Study the drawing (mm; zero at the part's minimum x, y, z) and answer. Give positions to 0.01 mm unless a question says otherwise; leave off trailing zeros. Order: outer loops, then holes, each group sorted by start corner. A loop starts at its lowest first (then second) coordinate and runs counter-clockwise, first axis right, second up. Notation, with made-up numbers: (55.5, -2.5) - (99.5, -2.5) arc R32 cw to (99.5, 31.5) - close; hole circle Ø4 at (-5, -7). An arc over 180 degrees is marked (long way). Write each question's results on one line, items separated by ' | '. Start each with the question number.
1. Determine the mould class of the marked faces 1, 2 and 3 for opening direction X: released by +X, released by -X, zero draft, split by the parting line, or undercut.
2. Section C-C (z = 9.5) is taken. Give the vertices of the cut face in (x, y), and give its area (3 significant figures).
3. Find the intervals of material crossed by L1, parallel to Y at x = 6, z = 9.4; L2, parallel to Y at x = 6, z = 6; L3, parallel to Z at x = 8, y = 8.5, in increasing order.
4. Section D-D (x = 3.75) is taken. Give the vertices of the cut face in (y, z).
5. Section B-B (x = 6) is taken. Give the vertices of the cut face in (y, z).
6. Section A-A (y = 6) is taken. Give the vertices of the cut face in (x, z), and give its area (3 significant figures).
7. Flat-ended cylindrical pins translate along their axes: pin 1 (1 mm diameter, centred on x = 4.5, z = 6, fed in from -Y); pin 2 (1.5 mm diameter, centred on x = 7, y = 6, fed in from -Z). Find the tip coordinate at first contact, or state that the pin passes through.
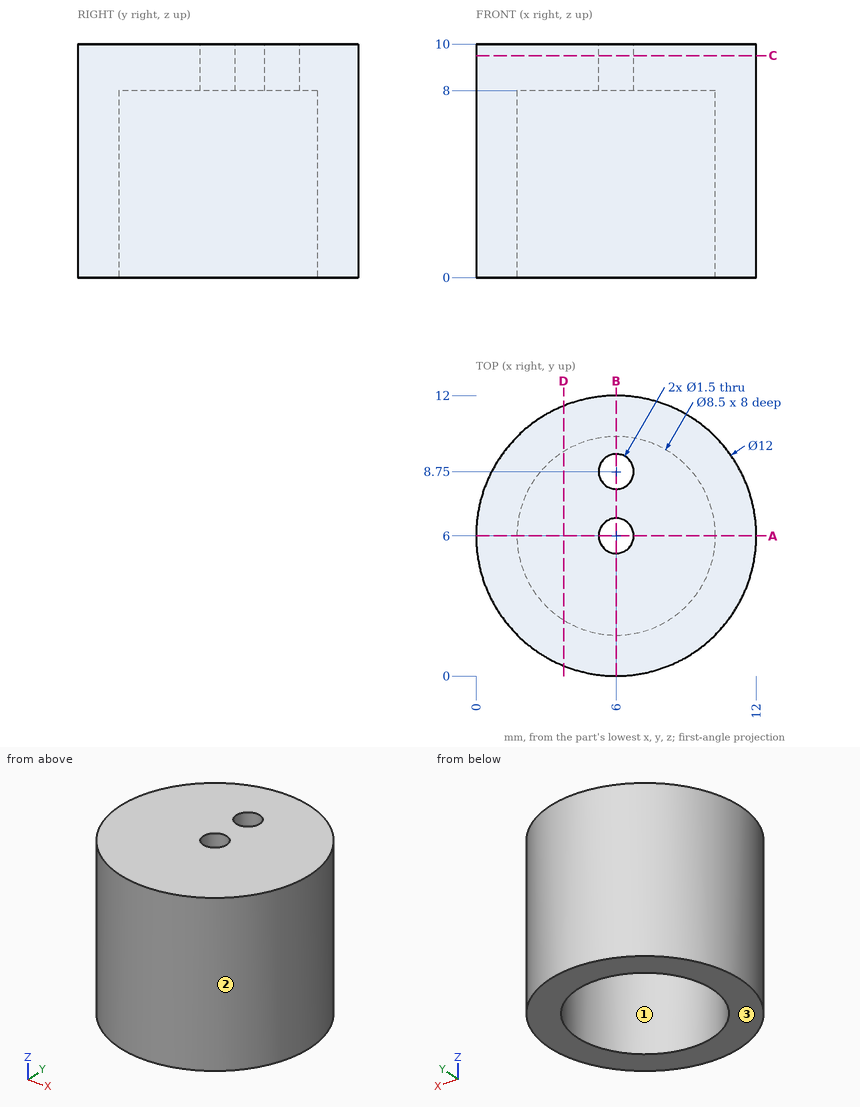
Reported:
1) face 1: undercut | face 2: split by the parting line | face 3: zero draft
2) outline: circle Ø12 at (6, 6); hole circle Ø1.5 at (6, 6); hole circle Ø1.5 at (6, 8.75) | area: 110 mm²
3) L1: 0 to 5.25, 6.75 to 8, 9.5 to 12 | L2: 0 to 1.75, 10.25 to 12 | L3: 8 to 10
4) outline: (0.44, 0) - (2.39, 0) - (2.39, 8) - (9.61, 8) - (9.61, 0) - (11.56, 0) - (11.56, 10) - (0.44, 10) - close
5) outline: (0, 0) - (1.75, 0) - (1.75, 8) - (5.25, 8) - (5.25, 10) - (0, 10) - close; (6.75, 8) - (8, 8) - (8, 10) - (6.75, 10) - close; (9.5, 8) - (10.25, 8) - (10.25, 0) - (12, 0) - (12, 10) - (9.5, 10) - close
6) outline: (0, 0) - (1.75, 0) - (1.75, 8) - (5.25, 8) - (5.25, 10) - (0, 10) - close; (6.75, 8) - (10.25, 8) - (10.25, 0) - (12, 0) - (12, 10) - (6.75, 10) - close | area: 49.0 mm²
7) pin 1: y = 0.08 | pin 2: z = 8
